Autodesk Inventor part; units mm, degrees
ref_plane "YZ Plane" through (0, 0, 0) normal (1, 0, 0) x (0, 1, 0)
ref_plane "XZ Plane" through (0, 0, 0) normal (0, 1, 0) x (-1, 0, 0)
ref_plane "XY Plane" through (0, 0, 0) normal (0, 0, 1) x (1, 0, 0)
sketch "Sketch1" plane through (0, 0, 0) normal (0, 0, 1) x (1, 0, 0)
  line L0 (169.1393, 4.2882) -> (221.6393, 4.2882)
  line L1 (221.6393, 4.2882) -> (221.6393, -32.0118)
  line L2 (221.6393, -32.0118) -> (169.1393, -32.0118)
  line L3 (169.1393, -32.0118) -> (169.1393, 4.2882)
  line L4 (-58.3607, 4.2882) -> (-17.8607, 4.2882)
  line L5 (-17.8607, 4.2882) -> (-17.8607, -32.0118)
  line L6 (-17.8607, -32.0118) -> (-58.3607, -32.0118)
  line L7 (-58.3607, -32.0118) -> (-58.3607, 4.2882)
  circle A0 centre (-58.3607, 4.2882) radius 12.5
  circle A1 centre (-58.3607, -32.0118) radius 12.5
  circle A2 centre (-17.8607, -32.0118) radius 12.5
  circle A3 centre (-17.8607, 4.2882) radius 12.5
  circle A4 centre (169.1393, 4.2882) radius 12.5
  circle A5 centre (169.1393, -32.0118) radius 12.5
  circle A6 centre (221.6393, -32.0118) radius 12.5
  circle A7 centre (221.6393, 4.2882) radius 12.5
  line L8 (-34.8317, -10.7118) -> (176.5512, -10.7118)
  line L9 (176.5512, -10.7118) -> (176.5512, -17.0118)
  line L10 (176.5512, -17.0118) -> (-34.8317, -17.0118)
  line L11 (-34.8317, -17.0118) -> (-34.8317, -10.7118)
  dimension "d0" = 36.3
  dimension "d1" = 40.5
  dimension "d2" = 52.5
  dimension "d3" = 239.5
  dimension "d4" = 25
  dimension "d5" = 15
  dimension "d6" = 15
extrude "Extrusion1" add sketch "Sketch1" along normal blind 2
sketch "Sketch2" plane through (0, 0, 2) normal (0, 0, 1) x (1, 0, 0)
  circle A0 centre (-58.3607, 4.2882) radius 5
  circle A1 centre (-58.3607, -32.0118) radius 5
  circle A2 centre (-17.8607, -32.0118) radius 5
  circle A3 centre (-17.8607, 4.2882) radius 5
  circle A4 centre (169.1393, 4.2882) radius 5
  circle A5 centre (169.1393, -32.0118) radius 5
  circle A6 centre (221.6393, -32.0118) radius 5
  circle A7 centre (221.6393, 4.2882) radius 5
  arc A8 (-45.8607, 4.2882) -> (-58.3607, -8.2118) centre (-58.3607, 4.2882) ccw
  arc A9 (-17.8607, -8.2118) -> (-30.3607, 4.2882) centre (-17.8607, 4.2882) ccw
  arc A10 (-58.3607, -19.5118) -> (-45.8607, -32.0118) centre (-58.3607, -32.0118) ccw
  arc A11 (-30.3607, -32.0118) -> (-17.8607, -19.5118) centre (-17.8607, -32.0118) ccw
  arc A12 (169.1393, -19.5118) -> (181.6393, -32.0118) centre (169.1393, -32.0118) ccw
  arc A13 (181.6393, 4.2882) -> (169.1393, -8.2118) centre (169.1393, 4.2882) ccw
  arc A14 (221.6393, -8.2118) -> (209.1393, 4.2882) centre (221.6393, 4.2882) ccw
  arc A15 (209.1393, -32.0118) -> (221.6393, -19.5118) centre (221.6393, -32.0118) ccw
  point P0 (0, 0)
  dimension "d9" = 10
extrude "Extrusion2" cut sketch "Sketch2" against normal blind 2
equation "\"d6\" = d5"
properties part number "NerfMount"
Build history of the part. All positions in model axes, mm. Round coordinates to 2 decimals unless told otherwise and drop trailing zeros. Order: outer loops, then holes, each group sorted by start corner. A loop starts at its lowest first (then second) coordinate and runs counter-clockwise, first axis right, second up. Notation, with made-up numbers: (67, -30.75) - (110, -30.75) arc R23 cw to (110, 6.25) - close; hole circle Ø9 at (-11, 23.25). An arc over 180 degrees is marked (long way). Use a Markdown table: item, result.
1) Pull direction X, two halves, no side cores. Call faces 1 (the face through (160.6, -41.14, 0.99)), 2 (the face through (-66.9, -41.14, 0.99)), 3 (the face through (80, -13, 0)): pulls with the +X half, pulls with the -X half, needs draft (parallel to the pull), parting line crosses it, or undercut.
Recorded:
| item | result |
|---|---|
| face 1 | undercut |
| face 2 | undercut |
| face 3 | needs draft |
2) Saw through at C-C on x = 114. Write the cut outline in (y, z), and give its area (3 significant figures).
Recorded:
| item | result |
|---|---|
| outline | (-17.01, 0) - (-10.71, 0) - (-10.71, 2) - (-17.01, 2) - close |
| area | 12.6 mm² |
3) Saw through at D-D on x = 203.5. Write the cut outline in (y, z), and give its area (3 significant figures).
Recorded:
| item | result |
|---|---|
| outline | (-32.01, 0) - (4.29, 0) - (4.29, 2) - (-32.01, 2) - close |
| area | 72.6 mm² |
4) Wall check: L1, parallel to Y at x = -7.5, z = 1.8; L2, parallel to Y at x = 167, z = 1.7; L3, parallel to X at y = -18, z = 0.95. Give the ranges that are in metal, low to high.
Recorded:
| item | result |
|---|---|
| L1 | y = -39.01 to -25.02, -17.01 to -10.71, -2.71 to 11.28 |
| L2 | y = -44.33 to -36.53, -27.49 to -19.7, -17.01 to -10.71, -8.03 to -0.23, 8.81 to 16.6 |
| L3 | x = -58.36 to -17.86, 169.14 to 221.64 |
5) Saw through at B-B on y = -22.5. Write the cut outline in (x, z).
Recorded:
| item | result |
|---|---|
| outline | (-66.47, 0) - (-9.75, 0) - (-9.75, 2) - (-66.47, 2) - close; (161.03, 0) - (229.75, 0) - (229.75, 2) - (161.03, 2) - close |
6) Flat gauge pins, fed straight in: pin 1 Ø1 at (x, z) = (-39, 1.5) entering from -Y; pin 2 Ø9 at (x, y) = (169.14, -32.01) entering from +Z; pin 3 Ø1 at (y, z) = (-10, 1) entering from -X; pin 4 Ø1 at (x, z) = (-40.5, 1) entering from +Y. Where does each tip first touch, or does it go through?
Recorded:
| item | result |
|---|---|
| pin 1 | stops at y = -32.01 |
| pin 2 | passes through |
| pin 3 | stops at x = -58.36 |
| pin 4 | stops at y = 4.29 |
7) Saw through at A-A on z = 1.7. Give the number of separate pieces and of enclosed holes in the cut face, and give its area (3 significant figures).
Recorded:
| item | result |
|---|---|
| separate pieces | 1 |
| enclosed holes | 8 |
| area | 6,870 mm² |
